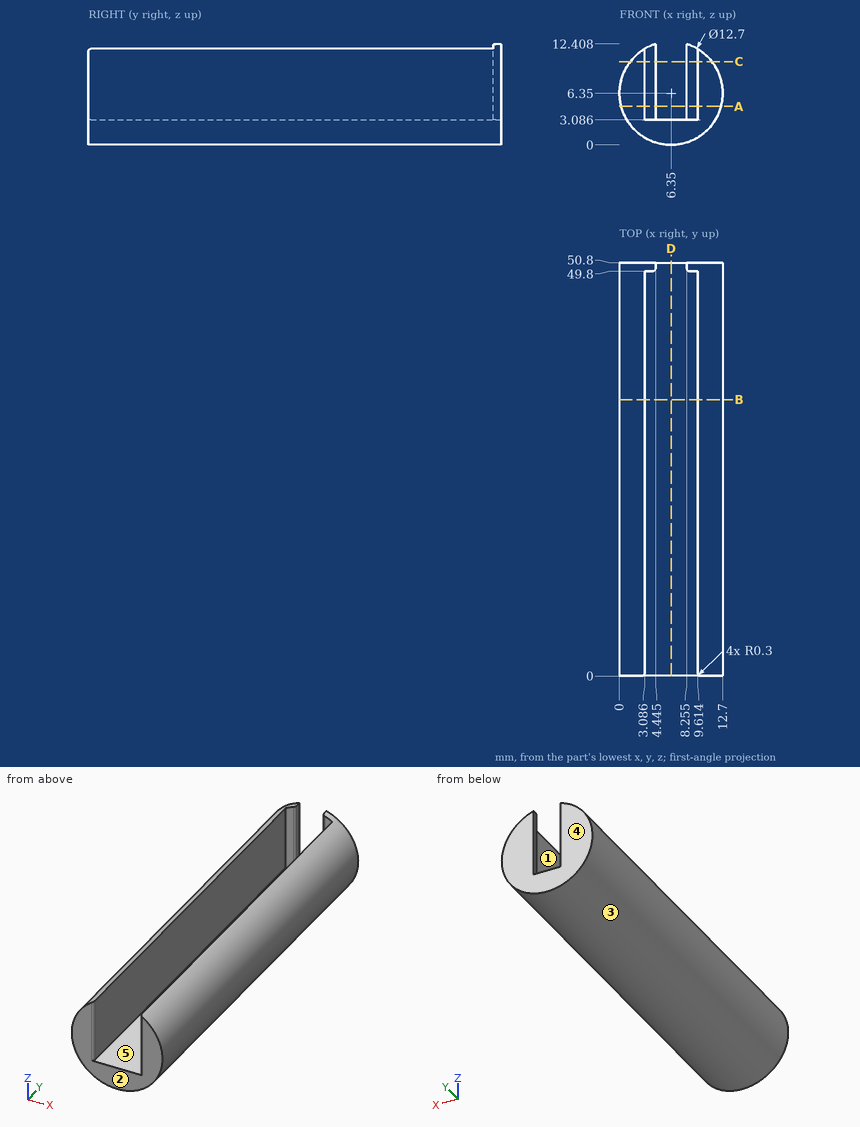
Can you work these out from the drawing? Everything is in mm from the part's minimum corner. A direction names the side the tool comes from. Round coordinates to 2 decimals unless told otherwise and drop trailing zeros. Loops run counter-clockwise (first coordinate to the right, second up) from the corner with the lowest first, then second, coordinate; pieces in that order, holes last. Notation, with made-up numbers: (56, 81) -> (102, 81) arc R18 ccw to (102, 98) -> close; hole circle Ø3 at (29.25, 18). An arc over 180 degrees is marked (long way). Answer in a Markdown table with one row per item.
Item 1: Will these pins go through, and if not, where does the flat tip stop? P1, Ø6, axis at y = 13.5, z = 3, coming from the -X side; P2, Ø3, axis at y = 33.5, z = 8, coming from the +X side; P3, Ø5, axis at y = 25.5, z = 11, coming from the -X side (1 decimal).
Answer block:
| item | result |
|---|---|
| P1 | x = 0.01 |
| P2 | x = 12.7 |
| P3 | x = 0.4 |
Item 2: Suppose I cut it at D-D, the plane x = 6.35. List the corners of the cut face in (y, z) for me.
Answer block:
| item | result |
|---|---|
| outline | (0, 0) -> (50.8, 0) -> (50.8, 3.09) -> (0, 3.09) -> close |
Item 3: If I drill on probe 1 along Y at (x, z) = (9, 10); probe 2 along X at (y, z) = (28, 9.25) (1 decimal); probe 3 along Z at (x, y) = (6.25, 19), over which ranges is the centre line in solid material (lowest first)?
Answer block:
| item | result |
|---|---|
| probe 1 | 49.8 to 50.8 |
| probe 2 | 0.7 to 3.1, 9.6 to 12 |
| probe 3 | 0 to 3.09 |
Item 4: Suppose I cut it at A-A, the plane z = 4.75. List the corners of the cut face in (x, y) for me (1 decimal).
Answer block:
| item | result |
|---|---|
| outline | (0.2, 0) -> (2.8, 0) arc R0.3 ccw to (3.1, 0.3) -> (3.1, 49.8) -> (4.1, 49.8) arc R0.3 ccw to (4.4, 50.1) -> (4.4, 50.8) -> (0.2, 50.8) -> close; (8.3, 50.1) arc R0.3 ccw to (8.6, 49.8) -> (9.6, 49.8) -> (9.6, 0.3) arc R0.3 ccw to (9.9, 0) -> (12.5, 0) -> (12.5, 50.8) -> (8.3, 50.8) -> close |
Item 5: Suppose I cut it at C-C, the plane z = 10.25. List the corners of the cut face in (x, y) for me (1 decimal).
Answer block:
| item | result |
|---|---|
| outline | (1.3, 0) -> (2.8, 0) arc R0.3 ccw to (3.1, 0.3) -> (3.1, 49.8) -> (4.1, 49.8) arc R0.3 ccw to (4.4, 50.1) -> (4.4, 50.8) -> (1.3, 50.8) -> close; (8.3, 50.1) arc R0.3 ccw to (8.6, 49.8) -> (9.6, 49.8) -> (9.6, 0.3) arc R0.3 ccw to (9.9, 0) -> (11.4, 0) -> (11.4, 50.8) -> (8.3, 50.8) -> close |
Item 6: Suppose I cut it at B-B, the plane y = 34. List the corners of the cut face in (x, z) for me.
Answer block:
| item | result |
|---|---|
| outline | (3.09, 3.09) -> (3.09, 11.8) arc R6.35 ccw (long way) to (9.61, 11.8) -> (9.61, 3.09) -> close |
Item 7: On a 3-axis mill with a long thin cutter (end or side, diameter ignored), from which of +Z, -Z, +X, -X, +Y, -Y can I reach the whole of each face in a straight line? I mean the marked faces 1 and 2. Say none if no direction works.
Answer block:
| item | result |
|---|---|
| face 1 | +Z, -Y |
| face 2 | +Z, -Z, +X, -X, -Y |
Item 8: We'd pull the mould along X, two halves only. Please class the marked faces 3, 4 and 5: released by +X, released by -X, zero draft, split by the parting line, or undercut.
Answer block:
| item | result |
|---|---|
| face 3 | split by the parting line |
| face 4 | zero draft |
| face 5 | undercut |
